Geometry: final body of the model. Coordinates: model frame, mm. Face numbers are marked on the shaded views. A direction names the side the tool comes from. Coordinates: 2 decimals unless noted, no trailing zeros. Loops run counter-clockwise (first coordinate to the right, second up) from the corner with the lowest first, then second, coordinate; pieces in that order, holes last. Notation, with made-up numbers: (52.25, 1) -> (86.25, 1) arc R26 ccw to (86.25, 15) -> close; hole circle Ø9 at (-27, 64.5). An arc over 180 degrees is marked (long way). One line per item, written item: value. Start each with the question number.
Item 1: Contact query for flat-ended pins moving along their axis: pin 1 Ø3.5 at (y, z) = (-12.8, 70.8) entering from +X; pin 2 Ø4 at (y, z) = (-12.8, 37.8) entering from -X; pin 3 Ø1.5 at (y, z) = (-0.5, 37) entering from +X; pin 4 Ø1 at (x, y) = (15, -15.5) entering from +Z. Output: stop coordinate, or through.
Item 2: Ray query, probe 1 along Z at (x, y) = (14, -13); probe 2 along Y at (x, z) = (13.75, 37.8); probe 3 along Z at (x, y) = (0.5, -17). Return the intervals inside material, ascending. Write a range as from..to.
Item 3: Section query C-C on x = 25.5. Return loops of the section in (y, z).
Item 4: Section query B-B on y = -3.8. Return loops of the section in (x, z), then the cut area to 3 significant figures.
Item 5: Set-up query: the marked faces 1, 2, 3 and 4. Return all of +Z, -Z, +X, -X, +Y, -Y with unobstructed straight access to the full face (end or side cutting, diameter ignored); none if empty.
Item 6: Section query D-D on z = 61.8. Return loops of the section in (x, y), then the cut area to 3 significant figures.
Item 7: Section query A-A on z = 37.8. Return loops of the section in (x, y), then the cut area to 3 significant figures.
Autodesk Inventor part; units mm, degrees
ref_plane "РабПлоскость1" through (12.2, 0, 0) normal (1, 0, 0) x (0, 1, 0)
ref_plane "РабПлоскость2" through (12.2, -3.8, 30.8) normal (0, -1, 0) x (1, 0, 0)
ref_plane "XZ Plane" through (0, 0, 0) normal (0, 1, 0) x (-1, 0, 0)
sketch "Эскиз1" plane through (0, 0, 0) normal (0, 0, 1) x (1, 0, 0)
  circle A0 centre (0, 0) radius 12.2
  dimension "d0" = 24.4
extrude "Выдавливание1" add sketch "Эскиз1" along normal blind 30.8
ref_plane "РабПлоскость1" through (12.2, 0, 0) normal (1, 0, 0) x (0, 1, 0)
sketch "Эскиз2" plane through (12.2, 0, 0) normal (1, 0, 0) x (0, 1, 0)
  line L0 (12.2, 0) -> (12.2, 30.8)
  line L1 (12.2, 30.8) -> (-19.8, 30.8)
  line L2 (-19.8, 30.8) -> (-19.8, 76.8)
  line L3 (-19.8, 76.8) -> (12.2, 76.8)
  line L4 (12.2, 76.8) -> (12.2, 30.8)
  point P0 (0, 0)
  dimension "d3" = 46
  dimension "d4" = 32
extrude "Выдавливание2" add sketch "Эскиз2" against normal blind 23.2
sketch "Эскиз3" plane through (12.2, 0, 0) normal (1, 0, 0) x (0, 0, -1)
  circle A0 centre (-70.8, -12.8) radius 3.7
  line L0 (0, 0) -> (0, -12.8)
  line L1 (0, -12.8) -> (-70.8, -12.8)
  point P0 (-76.8, -19.8)
  dimension "d10" = 7.4
  dimension "d11" = 12.8
  dimension "d12" = 70.8
extrude "Выдавливание3" add sketch "Эскиз3" along normal blind 2
ref_plane "РабПлоскость2" through (12.2, -3.8, 30.8) normal (0, -1, 0) x (1, 0, 0)
mirror "Зеркальное отражение1" about plane through (12.2, -3.8, 30.8) normal (0, -1, 0) of "Выдавливание3"
sketch "Эскиз4" plane through (12.2, 0, 0) normal (1, 0, 0) x (0, 0, -1)
  line L0 (-30.8, -5.2764) -> (-30.8, -19.8)
  line L1 (-30.8, -19.8) -> (-37.8, -19.8)
  line L2 (-30.8, -19.8) -> (-76.8, -19.8)
  line L3 (-37.8, -19.8) -> (-37.8, -12.8)
  circle A0 centre (-37.8, -12.8) radius 3.7
  point P0 (0, 0)
  dimension "d15" = 7
  dimension "d16" = 7
  dimension "d17" = 7.4
extrude "Выдавливание4" add sketch "Эскиз4" along normal blind 2
mirror "Зеркальное отражение2" about plane through (12.2, -3.8, 30.8) normal (0, -1, 0) of "Выдавливание4"
sketch "Эскиз5" plane through (12.2, 0, 0) normal (1, 0, 0) x (0, 0, -1)
  circle A0 centre (-70.8, -12.8) radius 3.7
  circle A1 centre (-70.8, 5.2) radius 3.7
  line L0 (-76.8, -19.8) -> (-61.8, -19.8)
  line L1 (-61.8, -19.8) -> (-61.8, -3.8)
  circle A2 centre (-61.8, -3.8) radius 3
  point P0 (0, 0)
  dimension "d20" = 15
  dimension "d21" = 16
  dimension "d22" = 6
extrude "Выдавливание5" add sketch "Эскиз5" along normal blind 18.5 contours A2
sketch "Эскиз6" plane through (14.2, -12.8, 70.8) normal (1, 0, 0) x (0, 0, -1)
  circle A0 centre (0, 0) radius 3.7
  circle A1 centre (0, 0) radius 1.5
  point P0 (70.8, 12.8)
  dimension "d25" = 3
extrude "Выдавливание6" cut sketch "Эскиз6" against normal blind 2 contours A1
mirror "Зеркальное отражение3" about plane through (12.2, -3.8, 30.8) normal (0, -1, 0) of "Выдавливание6"
sketch "Эскиз8" plane through (14.2, -12.8, 37.8) normal (1, 0, 0) x (0, 0, -1)
  circle A0 centre (0, 0) radius 3.7
  circle A1 centre (0, 0) radius 1.5
  point P0 (37.8, 12.8)
  dimension "d28" = 3
extrude "Выдавливание7" cut sketch "Эскиз8" against normal blind 2 contours A1
mirror "Зеркальное отражение4" about plane through (12.2, -3.8, 30.8) normal (0, -1, 0) of "Выдавливание7"
sketch "Эскиз9" plane through (12.2, 0, 0) normal (1, 0, 0) x (0, 0, -1)
  circle A0 centre (-61.8, -3.8) radius 3
  circle A1 centre (-61.8, -3.8) radius 5
  point P0 (0, 0)
  dimension "d31" = 10
extrude "Выдавливание8" add sketch "Эскиз9" along normal blind 2
properties part number "Мотор"
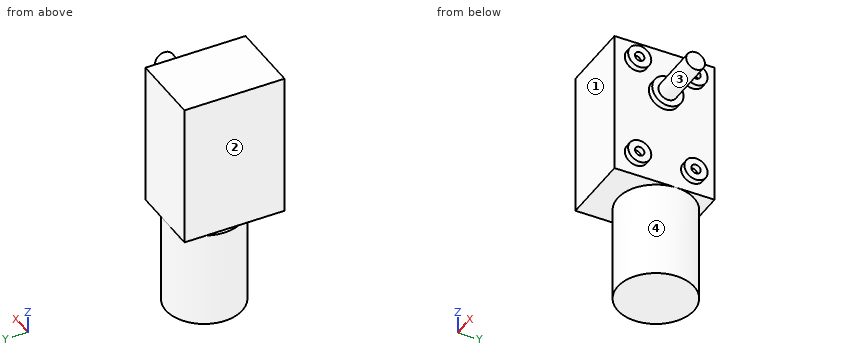
Reply:
1. pin 1: stops at x = 14.2
1. pin 2: stops at x = -11
1. pin 3: stops at x = 12.2
1. pin 4: passes through
2. probe 1: z = 34.11..36.31, 39.29..41.49, 67.11..69.31, 72.29..74.49
2. probe 2: y = -16.5..-14.3, -11.3..-9.1, 1.5..3.7, 6.7..8.9
2. probe 3: z = 30.8..76.8
3. outline: circle Ø6 at (-3.8, 61.8)
4. outline: (-11.59, 0) -> (11.59, 0) -> (11.59, 30.8) -> (12.2, 30.8) -> (12.2, 56.8) -> (14.2, 56.8) -> (14.2, 58.8) -> (30.7, 58.8) -> (30.7, 64.8) -> (14.2, 64.8) -> (14.2, 66.8) -> (12.2, 66.8) -> (12.2, 76.8) -> (-11, 76.8) -> (-11, 30.8) -> (-11.59, 30.8) -> close
4. area: 1,900 mm²
5. face 1: +Z, -Z, +X, -X, -Y
5. face 2: +Z, -X, +Y, -Y
5. face 3: +X
5. face 4: -Z
6. outline: (-11, -19.8) -> (12.2, -19.8) -> (12.2, -8.8) -> (14.2, -8.8) -> (14.2, -6.8) -> (30.7, -6.8) -> (30.7, -0.8) -> (14.2, -0.8) -> (14.2, 1.2) -> (12.2, 1.2) -> (12.2, 12.2) -> (-11, 12.2) -> close
6. area: 861 mm²
7. outline: (-11, -19.8) -> (12.2, -19.8) -> (12.2, -16.5) -> (14.2, -16.5) -> (14.2, -14.3) -> (12.2, -14.3) -> (12.2, -11.3) -> (14.2, -11.3) -> (14.2, -9.1) -> (12.2, -9.1) -> (12.2, 1.5) -> (14.2, 1.5) -> (14.2, 3.7) -> (12.2, 3.7) -> (12.2, 6.7) -> (14.2, 6.7) -> (14.2, 8.9) -> (12.2, 8.9) -> (12.2, 12.2) -> (-11, 12.2) -> close
7. area: 760 mm²
